from build123d import *

# Parameters (mm, degrees)
SKETCH1_W           = 45
SKETCH1_H           = 36
BOSS_EXTRUDE1_DEPTH = 3
SKETCH2_W           = 10
SKETCH2_H           = 10
BOSS_EXTRUDE2_DEPTH = 5
SKETCH2_3_R         = 5
BOSS_EXTRUDE3_DEPTH = 27


with BuildPart() as part:
    # Sketch1 → Boss-Extrude1 (new body)
    with BuildSketch(Plane(origin=(0, 0, 0), x_dir=(1, 0, 0), z_dir=(0, 1, 0))):
        Rectangle(SKETCH1_W, SKETCH1_H)
    extrude(amount=BOSS_EXTRUDE1_DEPTH)

    # Sketch2 → Boss-Extrude2 (add)
    with BuildSketch(Plane(origin=(0, 3, 0), x_dir=(1, 0, 0), z_dir=(0, 1, 0))):
        with BuildLine():
            ThreePointArc((17.5, 5), (13.964466095, 3.535533907), (12.5, 4e-09))
            Line((12.5, 0), (22.5, 0))
            ThreePointArc((22.5, 0), (21.035533906, 3.535533906), (17.5, 5))
        make_face()
        with BuildLine():
            Line((22.5, 0), (12.5, 0))
            ThreePointArc((12.5, 4e-09), (13.964466099, -3.535533911), (17.500000019, -5))
            ThreePointArc((17.500000019, -5), (21.035533913, -3.535533899), (22.5, 0))
        make_face()
        with Locations((17.5, 0)):
            Rectangle(SKETCH2_W, SKETCH2_H)
    extrude(amount=BOSS_EXTRUDE2_DEPTH)

    # Sketch2<3> → Boss-Extrude3 (add)
    with BuildSketch(Plane(origin=(0, 3, 0), x_dir=(1, 0, 0), z_dir=(0, 1, 0))):
        with Locations(Location((17.5, 0, 0), (0, 0, 270))):
            Circle(SKETCH2_3_R)
    extrude(amount=BOSS_EXTRUDE3_DEPTH)


solid = part.part
Here's how the part is built. I have some questions about the finished solid (model axes, mm). A direction names the side the tool comes from. Coordinates: 2 decimals unless noted, no trailing zeros. Order: outer loops, then holes, each group sorted by start corner. A loop starts at its lowest first (then second) coordinate and runs counter-clockwise, first axis right, second up. Notation, with made-up numbers: M 77.25,38 L 133.25,38 A20 cw 133.25,72 Z; hole C 43.25,78 d11. An arc over 180 degrees is marked long. Answer as CSV lines item,"result". Start each with the question number.
1. I want a section at D-D, the plane z = -3.5. Write out the boundary of the cut face in (x, y), and give its area (3 significant figures).
2. For pin 1 (10 mm diameter, centred on y = 15.5, z = -9.5, fed in from -X); pin 2 (4 mm diameter, centred on x = 18.5, y = 6.5, fed in from -Z); pin 3 (10 mm diameter, centred on y = 21.5, z = 9.5, fed in from +X), each with a flat end and sliding along its axis, tell me the tip position at first contact or that it passes through.
3. I want a section at A-A, the plane z = 1. Write out the boundary of the cut face in (x, y).
4. I want a section at C-C, the plane x = 9. Write out the boundary of the cut face in (y, z), and give its area (3 significant figures).
5. On a 3-axis mill with a long thin cutter (end or side, diameter ignored), from which of +Z, -Z, +X, -X, +Y, -Y can I reach the whole of each face in a straight line? I mean faces 1 (the flat face through (14, 8, -4)), 2 (the flat face through (21, 8, -4)), 3 (the flat face through (17, 5, 5)), 4 (the flat face through (21, 8, 4)). Say none if no direction works.
6. I want a section at B-B, the plane y = 28. Write out the boundary of the cut face in (x, z).
7. I need wall thicknesses on line 1 (Y direction, x = -8, z = -14.5); line 2 (X direction, y = 4.75, z = -2); line 3 (Z direction, x = 16, y = 7). Which ranges of each line are inside material? Lowest first, please. Write a range as [from, to].
Recorded:
1,outline,"M -22.5,0 L 22.5,0 L 22.5,8 L 21.07,8 L 21.07,30 L 13.93,30 L 13.93,8 L 12.5,8 L 12.5,3 L -22.5,3 Z"
1,area,"342 mm2"
2,pin 1,"stops at x = 15.32"
2,pin 2,"stops at z = -5"
2,pin 3,"stops at x = 19.68"
3,outline,"M -22.5,0 L 22.5,0 L 22.5,8 L 22.4,8 L 22.4,30 L 12.6,30 L 12.6,8 L 12.5,8 L 12.5,3 L -22.5,3 Z"
4,outline,"M 0,-18 L 3,-18 L 3,18 L 0,18 Z"
4,area,"108 mm2"
5,face 1,"-Z, -X, +Y"
5,face 2,"-Z, +X, +Y"
5,face 3,"+Z, +X, -X, +Y"
5,face 4,"+Z, +X, +Y"
6,outline,"C 17.5,0 d10"
7,line 1,"y = [0, 3]"
7,line 2,"x = [12.5, 22.5]"
7,line 3,"z = [-5, 5]"
